from build123d import *

# Parameters (mm, degrees)
SKETCH1_R           = 76.2
SKETCH1_R_2         = 73.025
BOSS_EXTRUDE1_DEPTH = 76.2
SKETCH3_R           = 76.2
BOSS_EXTRUDE2_DEPTH = 3.175
SKETCH5_R           = 2.1828125
CUT_EXTRUDE2_DEPTH  = 4.175
SKETCH11_R          = 2.1828125
CUT_EXTRUDE11_DEPTH = 4.175
SKETCH12_R          = 18.984546406
CUT_EXTRUDE12_DEPTH = 4.175
CUT_EXTRUDE13_DEPTH = 4.175
CIRPATTERN1_COUNT   = 4


with BuildPart() as part:
    # Sketch1 → Boss-Extrude1 (new body)
    with BuildSketch(Plane.XY):
        Circle(SKETCH1_R)
        Circle(SKETCH1_R_2, mode=Mode.SUBTRACT)
    extrude(amount=BOSS_EXTRUDE1_DEPTH)

    # Sketch3 → Boss-Extrude2 (add)
    with BuildSketch(Plane.XY):
        Circle(SKETCH3_R)
    extrude(amount=BOSS_EXTRUDE2_DEPTH)

    # Sketch5 → Cut-Extrude2 (cut, through all)
    with BuildSketch(Plane.XY.offset(3.175)):
        with Locations((0, 37.81298)):
            Circle(SKETCH5_R)
        with Locations((37.81298, 0)):
            Circle(SKETCH5_R)
        with Locations((-37.81298, 0)):
            Circle(SKETCH5_R)
        with Locations((0, -37.81298)):
            Circle(SKETCH5_R)
    extrude(amount=-CUT_EXTRUDE2_DEPTH, mode=Mode.SUBTRACT)

    # Sketch11 → Cut-Extrude11 (cut, through all)
    with BuildSketch(Plane.XY.offset(3.175)):
        with Locations((-35.921024484, 35.921024484)):
            Circle(SKETCH11_R)
        with Locations((-35.921024484, -35.921024484)):
            Circle(SKETCH11_R)
        with Locations((35.921024484, -35.921024484)):
            Circle(SKETCH11_R)
        with Locations((35.921024484, 35.921024484)):
            Circle(SKETCH11_R)
    extrude(amount=-CUT_EXTRUDE11_DEPTH, mode=Mode.SUBTRACT)

    # Sketch12 → Cut-Extrude12 (cut, through all)
    with BuildSketch(Plane.XY.offset(3.175)):
        Circle(SKETCH12_R)
    extrude(amount=-CUT_EXTRUDE12_DEPTH, mode=Mode.SUBTRACT)

    # Sketch13 → Cut-Extrude13 (cut, through all)
    with BuildSketch(Plane.XY.offset(3.175)):
        with BuildLine():
            Line((-18.887713582, 26.073256792), (-33.213845797, 45.849548003))
            ThreePointArc((-33.213845797, 45.849548003), (-34.276091741, 50.925360779), (-31.200233714, 55.10044631))
            ThreePointArc((-31.200233714, 55.10044631), (-24.962317442, 58.192752772), (-18.42261337, 60.581524279))
            ThreePointArc((-18.42261337, 60.581524279), (-13.277568117, 59.932870951), (-10.331766338, 55.665026803))
            Line((-10.331766338, 55.665026803), (-5.875364286, 31.655023908))
            ThreePointArc((-5.875364286, 31.655023908), (-6.559884807, 27.42673862), (-9.773713061, 24.595083138))
            ThreePointArc((-9.773713061, 24.595083138), (-10.43339446, 24.322579255), (-11.085487572, 24.032385376))
            ThreePointArc((-11.085487572, 24.032385376), (-15.352183804, 23.65520096), (-18.887713582, 26.073256792))
        make_face()
        with BuildLine():
            Line((-45.533204085, 33.646217178), (-25.893361536, 19.133590161))
            ThreePointArc((-25.893361536, 19.133590161), (-23.508869462, 15.575337449), (-23.926411262, 11.312401411))
            ThreePointArc((-23.926411262, 11.312401411), (-24.511909026, 9.980475814), (-25.023328549, 8.618387895))
            ThreePointArc((-25.023328549, 8.618387895), (-27.702333545, 5.276248304), (-31.894176796, 4.395671802))
            Line((-31.894176796, 4.395671802), (-56.085574643, 7.729742659))
            ThreePointArc((-56.085574643, 7.729742659), (-60.4859006, 10.473713006), (-61.373317696, 15.582992084))
            ThreePointArc((-61.373317696, 15.582992084), (-58.645731892, 23.878691299), (-54.802742327, 31.720233302))
            ThreePointArc((-54.802742327, 31.720233302), (-50.598737942, 34.756446226), (-45.533204085, 33.646217178))
        make_face()
    cut_extrude13 = extrude(amount=-CUT_EXTRUDE13_DEPTH, mode=Mode.SUBTRACT)

    # CirPattern1: Cut-Extrude13 ×4 about axis
    cirpattern1_axis = Axis((0, 0, 0), (0, 0, 1))
    for i in range(1, CIRPATTERN1_COUNT):
        add(cut_extrude13.rotate(cirpattern1_axis, i * 360 / CIRPATTERN1_COUNT), mode=Mode.SUBTRACT)


solid = part.part
The listing builds one solid part. Answer for the finished solid, in the listing's coordinates (mm). Round coordinates to 2 decimals unless told otherwise and drop trailing zeros. Write each loop counter-clockwise with the first axis right and the second up, starting at its lowest first coordinate (ties: lowest second). Pieces come first, ordered by that corner, then holes. Notation, with made-up numbers: (-37.75, 9) - (21.25, 9) arc R16 cw to (21.25, 29) - close; hole circle Ø2 at (11, -14). An arc over 180 degrees is marked (long way). Use a Markdown table: item, result. Add a question column.
1. For a pull along X with two mould halves and no side action, classify faces 1 (the face through (16, -16, 0)), 2 (the face through (8.135, -43.828, 1.61)), 3 (the face through (-59.97, -13.34, 1.61)) as +X half, -X half, draft (parallel to the pull), parting line (faces both ways), or undercut.
2. The part is cut by section C-C (y = -50.5). Write down the section's boundary in (x, z) (3 decimals), and give its area (3 significant figures).
3. Flat-ended cylindrical pins translate along their axes: P1, Ø5.5, axis at x = 0, y = 37.81, coming from the -Z side; P2, Ø1, axis at y = -17, z = 20.5, coming from the -X side; P3, Ø3, axis at y = -17.5, z = 67, coming from the +X side; P4, Ø1.5, axis at x = 57.5, z = 57, coming from the -Y side. Find the tip coordinate at first contact, or state that the pin passes through.
4. The part is cut by section A-A (x = 0). Write down the section's boundary in (y, z) (3 decimals).
5. The part is cut by section D-D (z = 65.5). Write down the section's boundary in (x, y) (3 decimals), and give its area (3 significant figures).
6. Consider line 1 (Y direction, x = 0, z = 2); line 2 (Z direction, x = 28, y = -3) (3 decimals); line 3 (X direction, y = -65, z = 70). Determine where each line is inside the solid, lowest interval first.
Reported:
| question | item | result |
|---|---|---|
| 1 | face 1 | draft |
| 1 | face 2 | undercut |
| 1 | face 3 | undercut |
| 2 | outline | (-57.063, 0) - (-34.776, 0) - (-34.776, 3.175) - (-52.748, 3.175) - (-52.748, 76.2) - (-57.063, 76.2) - close; (-6.96, 0) - (9.373, 0) - (9.373, 3.175) - (-6.96, 3.175) - close; (34.354, 0) - (57.063, 0) - (57.063, 76.2) - (52.748, 76.2) - (52.748, 3.175) - (34.354, 3.175) - close |
| 2 | area | 825 mm^2 |
| 3 | P1 | z = 0 |
| 3 | P2 | x = -74.39 |
| 3 | P3 | x = 74.5 |
| 3 | P4 | y = -50.85 |
| 4 | outline | (-76.2, 0) - (-39.996, 0) - (-39.996, 3.175) - (-73.025, 3.175) - (-73.025, 76.2) - (-76.2, 76.2) - close; (-35.63, 0) - (-18.985, 0) - (-18.985, 3.175) - (-35.63, 3.175) - close; (18.985, 0) - (35.63, 0) - (35.63, 3.175) - (18.985, 3.175) - close; (39.996, 0) - (76.2, 0) - (76.2, 76.2) - (73.025, 76.2) - (73.025, 3.175) - (39.996, 3.175) - close |
| 5 | outline | circle Ø152.4 at (0, 0); hole circle Ø146.05 at (0, 0) |
| 5 | area | 1,490 mm^2 |
| 6 | line 1 | -76.2 to -40, -35.63 to -18.98, 18.98 to 35.63, 40 to 76.2 |
| 6 | line 2 | 0 to 3.175 |
| 6 | line 3 | -39.77 to -33.28, 33.28 to 39.77 |
